Can you work these out from the model? Positions are in its coordinate system, mm. Face numbers are marked on the shaded views. A direction names the side the tool comes from. Round coordinates to 2 decimals unless told otherwise and drop trailing zeros. Write each loop counter-clockwise with the first axis right and the second up, starting at its lowest first coordinate (ties: lowest second). Pieces come first, ordered by that corner, then holes.
Q1. If we section it at B-B (x = 0): Please give me the cut outline in (y, z) (1 decimal), plus the area to 3 significant figures.
Q2. Please list where these lines run through material, in increasing order: line 1 along Y through (x, z) = (0, 0.7) (3 decimals); line 2 along X through (y, z) = (-1.5, 0.8) (3 decimals); line 3 along X through (y, z) = (2.5, 0.95) (1 decimal).
Q3. For the marked faces 1 and 2, which set-ups out of +Z, -Z, +X, -X, +Y, -Y let a thin tool reach every point of the face, with its end or its side?
Q4. If we section it at C-C (z = 0.8): Give the number of separate pieces and of enclosed holes in the cut face, plus the area to 3 significant figures.
Q5. If we section it at D-D (y = 0): Please give me the cut outline in (x, z) (1 decimal).
Q6. I'm going to push flat-ended pins straight in: pin 1 Ø0.5 at (y, z) = (-2.5, 0.5) entering from +X (3 decimals); pin 2 Ø0.5 at (x, z) = (2.5, 0.5) entering from +Y; pin 3 Ø0.8 at (y, z) = (5.5, 0.5) entering from -X (3 decimals). Where does each tip first touch, or does it pass through?
Q7. We'd pull the mould along X, two halves only. Please class the marked faces 3, 4 and 5: +X half, -X half, draft (parallel to the pull), parting line (faces both ways), or undercut.
from build123d import *

# Parameters (mm, degrees)
BOSS_EXTRUDE1_DEPTH = 1.5875
FILLET1_R           = 2.54
SKETCH2_R           = 3.175
CUT_EXTRUDE1_DEPTH  = 27.229804731


with BuildPart() as part:
    # Sketch1 → Boss-Extrude1 (new body)
    with BuildSketch(Plane.XY):
        with BuildLine():
            Line((-5.175, 15.370071332), (-5.175, -5.175))
            Line((-5.175, -5.175), (5.175, -5.175))
            Line((5.175, -5.175), (5.175, 15.370071332))
            ThreePointArc((5.175, 15.370071332), (0, 25.4), (-5.175, 15.370071332))
        make_face()
        Polygon((-3.175, -1.5875), (-3.175, 1.5875), (-1.5875, 1.5875), (-1.5875, 3.175), (1.5875, 3.175), (1.5875, 1.5875), (3.175, 1.5875), (3.175, -1.5875), (1.5875, -1.5875), (1.5875, -3.175), (-1.5875, -3.175), (-1.5875, -1.5875), align=None, mode=Mode.SUBTRACT)
    extrude(amount=BOSS_EXTRUDE1_DEPTH)

    # Fillet1
    fillet1_edges = [part.edges().sort_by_distance(p)[0] for p in [
        (5.175, -5.175, 0.79375),
        (-5.175, -5.175, 0.79375),
    ]]
    fillet(fillet1_edges, radius=FILLET1_R)

    # Sketch2 → Cut-Extrude1 (cut, through all)
    with BuildSketch(Plane.XY.offset(1.5875)):
        with Locations((0, 19.05)):
            Circle(SKETCH2_R)
    extrude(amount=-CUT_EXTRUDE1_DEPTH, mode=Mode.SUBTRACT)


solid = part.part
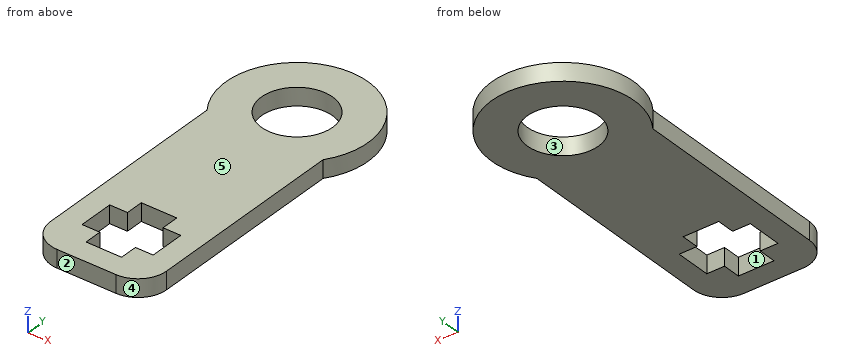
A:
1. outline: (-5.2, 0) - (-3.2, 0) - (-3.2, 1.6) - (-5.2, 1.6) - close; (3.2, 0) - (15.9, 0) - (15.9, 1.6) - (3.2, 1.6) - close; (22.2, 0) - (25.4, 0) - (25.4, 1.6) - (22.2, 1.6) - close
1. area: 28.4 mm2
2. line 1: y = -5.175 to -3.175, 3.175 to 15.875, 22.225 to 25.4
2. line 2: x = -5.175 to -3.175, 3.175 to 5.175
2. line 3: x = -5.2 to -1.6, 1.6 to 5.2
3. face 1: +Z, -Z
3. face 2: +Z, -Z, +X, -X, -Y
4. separate pieces: 1
4. enclosed holes: 2
4. area: 255 mm2
5. outline: (-5.2, 0) - (-3.2, 0) - (-3.2, 1.6) - (-5.2, 1.6) - close; (3.2, 0) - (5.2, 0) - (5.2, 1.6) - (3.2, 1.6) - close
6. pin 1: stops at x = 5.175
6. pin 2: stops at y = 24.99
6. pin 3: stops at x = -5.175
7. face 3: undercut
7. face 4: +X half
7. face 5: draft
